The model under review builds one solid part; all positions refer to its coordinate system, in mm. A direction names the side the tool comes from. Coordinates: 2 decimals unless noted, no trailing zeros. Write each loop counter-clockwise with the first axis right and the second up, starting at its lowest first coordinate (ties: lowest second). Pieces come first, ordered by that corner, then holes. Notation, with made-up numbers: (49, -31) - (82, -31) arc R19 ccw to (82, -16) - close; hole circle Ø11 at (8, -15.75). An arc over 180 degrees is marked (long way). Return JSON: item names as keys, results as strings. Group by question number.
(1) For pin 1 Ø4 at (y, z) = (15.5, -5) entering from -X; pin 2 Ø1.5 at (y, z) = (12, -19) entering from -X; pin 3 Ø1 at (x, z) = (8.5, -21.5) entering from -Y, all flat-tipped, find the tip position at first contact; note any pin that passes through.
(2) We need section A-A on z = 7.7. State the section outline as (x, y) points.
(3) Draft analysis for pull direction Z (two halves, no side actions). For faces 4 (the face through (3.46, -10.73, 9.9)), 5 (the face through (0.867, -3.905, -37.042)), 6 (the face through (-1.57, 10.609, 11.487)), 7 (the face through (0, 0, 0)), state which applies: released by +Z, released by -Z, zero draft, split by the parting line, or undercut.
(4) To check wall thickness, follow L1, parallel to Z at x = -4, y = 2; L2, parallel to X at y = 9.75, z = 7.7; L3, parallel to X at y = -10.5, z = 7.7. State the ranges of each line that lie inside material, in increasing order. Write a range as from..to.
(5) Tool access review of faces 1 (the face through (-6.92, 13.31, 7.49)), 2 (the face through (4, -7, 15.2)), 3 (the face through (0, 0, -34)): name each direction out of +Z, -Z, +X, -X, +Y, -Y from which nothing blocks a thin tool from reaching the whole face with its end or side.
```python
from build123d import *

# Parameters (mm, degrees)
SKETCH_1_R               = 15
SKETCH_1_R_2             = 7.55
EXTRUDE_1_DEPTH          = 15.2
CUT_EXTRUDE_1_DEPTH      = 27.096743092
CUT_EXTRUDE_1_DEPTH_BACK = 27.096743092
SKETCH_2_R               = 4.1
SKETCH_8_R               = 4
CUT_EXTRUDE_2_DEPTH      = 6


with BuildPart() as part:
    # 스케치1 → 보스-돌출1 (new body)
    with BuildSketch(Plane.XY):
        with Locations(Location((0, 0, 0), (0, 0, 180))):
            Circle(SKETCH_1_R)
        with Locations(Location((0, 0, 0), (0, 0, 180))):
            Circle(SKETCH_1_R_2, mode=Mode.SUBTRACT)
    extrude(amount=EXTRUDE_1_DEPTH)

    # 스케치2 → 컷-돌출1 (cut, two sides: drawn at the far end of the back side and taken through both)
    with BuildSketch(Plane(origin=(0, 0, 0), x_dir=(1, 0, 0), z_dir=(0, 1, 0)).offset(-CUT_EXTRUDE_1_DEPTH_BACK)):
        with Locations(Location((0, -7.7, 0), (0, 0, 270))):
            Circle(SKETCH_2_R)
    extrude(amount=CUT_EXTRUDE_1_DEPTH + CUT_EXTRUDE_1_DEPTH_BACK, mode=Mode.SUBTRACT)

    # 스케치3 for 로프트4 → 로프트4 section 0
    with BuildSketch(Plane.XY):
        with BuildLine():
            # circular arc as an exact rational Bezier (weights 1, cos(half-angle), 1)
            Bezier((8, -13.856406461), (16.000000001, -9.237604308), (16, 0), weights=[1, 0.866025404, 1])
            Bezier((16, 0), (16.000000001, 9.237604308), (8, 13.856406461), weights=[1, 0.866025404, 1])
            Bezier((8, 13.856406461), (0, 18.475208613), (-8, 13.856406461), weights=[1, 0.866025404, 1])
            Bezier((-8, 13.856406461), (-16.000000001, 9.237604308), (-16, 0), weights=[1, 0.866025404, 1])
            Bezier((-16, 0), (-16.000000001, -9.237604308), (-8, -13.856406461), weights=[1, 0.866025404, 1])
            Bezier((-8, -13.856406461), (0, -18.475208613), (8, -13.856406461), weights=[1, 0.866025404, 1])
        make_face()
    # 스케치4 → 로프트4 section 1
    with BuildSketch(Plane.XY.offset(-15)):
        with BuildLine():
            Line((11.25, -19.485571585), (22.5, 0))
            Line((22.5, 0), (11.25, 19.485571585))
            Line((11.25, 19.485571585), (-11.25, 19.485571585))
            Line((-11.25, 19.485571585), (-22.5, 0))
            Line((-22.5, 0), (-11.25, -19.485571585))
            Line((-11.25, -19.485571585), (11.25, -19.485571585))
        make_face()
    loft()

    # 로프트5: read off the stored shape, not the designer's step
    # 로프트5: loft between two sections, ruled curve by curve
    loft_5_from = [
        Edge.make_bspline([(22.5, 0, -15), (20.625, -3.247595264, -15), (18.75, -6.495190528, -15), (15, -12.990381057, -15), (13.125, -16.237976321, -15), (11.25, -19.485571585, -15)], [0, 0, 0, 0, 0.5, 0.5, 1, 1, 1, 1], 3),
        Edge.make_bspline([(11.25, -19.485571585, -15), (7.5, -19.485571585, -15), (3.75, -19.485571585, -15), (-3.75, -19.485571585, -15), (-7.5, -19.485571585, -15), (-11.25, -19.485571585, -15)], [0, 0, 0, 0, 0.5, 0.5, 1, 1, 1, 1], 3),
        Edge.make_bspline([(11.25, 19.485571585, -15), (13.125, 16.237976321, -15), (15, 12.990381057, -15), (18.75, 6.495190528, -15), (20.625, 3.247595264, -15), (22.5, 0, -15)], [0, 0, 0, 0, 0.5, 0.5, 1, 1, 1, 1], 3),
        Edge.make_bspline([(-11.25, -19.485571585, -15), (-13.125, -16.237976321, -15), (-15, -12.990381057, -15), (-18.75, -6.495190528, -15), (-20.625, -3.247595264, -15), (-22.5, 0, -15)], [0, 0, 0, 0, 0.5, 0.5, 1, 1, 1, 1], 3),
        Edge.make_bspline([(-22.5, 0, -15), (-20.625, 3.247595264, -15), (-18.75, 6.495190528, -15), (-15, 12.990381057, -15), (-13.125, 16.237976321, -15), (-11.25, 19.485571585, -15)], [0, 0, 0, 0, 0.5, 0.5, 1, 1, 1, 1], 3),
        Edge.make_bspline([(-11.25, 19.485571585, -15), (-7.5, 19.485571585, -15), (-3.75, 19.485571585, -15), (3.75, 19.485571585, -15), (7.5, 19.485571585, -15), (11.25, 19.485571585, -15)], [0, 0, 0, 0, 0.5, 0.5, 1, 1, 1, 1], 3),
    ]
    loft_5_to = [
        Edge.make_bspline([(5.352991825, 3.333635602, -40), (5.388078026, 2.283194817, -40), (5.423164227, 1.232754033, -40), (5.493336629, -0.868127536, -40), (5.52842283, -1.918568321, -40), (5.563509031, -2.969009106, -40)], [0, 0, 0, 0, 0.5, 0.5, 1, 1, 1, 1], 3),
        Edge.make_bspline([(5.563509031, -2.969009106, -40), (4.671343726, -3.524615039, -40), (3.779178422, -4.080220973, -40), (1.994847814, -5.19143284, -40), (1.10268251, -5.747038774, -40), (0.210517206, -6.302644707, -40)], [0, 0, 0, 0, 0.5, 0.5, 1, 1, 1, 1], 3),
        Edge.make_bspline([(-0.210517206, 6.302644707, -40), (0.716734299, 5.807809856, -40), (1.643985804, 5.312975006, -40), (3.498488815, 4.323305304, -40), (4.42574032, 3.828470453, -40), (5.352991825, 3.333635602, -40)], [0, 0, 0, 0, 0.5, 0.5, 1, 1, 1, 1], 3),
        Edge.make_bspline([(0.210517206, -6.302644707, -40), (-0.716734299, -5.807809856, -40), (-1.643985804, -5.312975006, -40), (-3.498488815, -4.323305304, -40), (-4.42574032, -3.828470453, -40), (-5.352991825, -3.333635602, -40)], [0, 0, 0, 0, 0.5, 0.5, 1, 1, 1, 1], 3),
        Edge.make_bspline([(-5.352991825, -3.333635602, -40), (-5.388078026, -2.283194817, -40), (-5.423164227, -1.232754033, -40), (-5.493336629, 0.868127536, -40), (-5.52842283, 1.918568321, -40), (-5.563509031, 2.969009106, -40)], [0, 0, 0, 0, 0.5, 0.5, 1, 1, 1, 1], 3),
        Edge.make_bspline([(-5.563509031, 2.969009106, -40), (-4.671343726, 3.524615039, -40), (-3.779178422, 4.080220973, -40), (-1.994847814, 5.19143284, -40), (-1.10268251, 5.747038774, -40), (-0.210517206, 6.302644707, -40)], [0, 0, 0, 0, 0.5, 0.5, 1, 1, 1, 1], 3),
    ]
    loft_5 = Solid(Shell([*[Face.make_surface_from_curves(loft_5_from[k], loft_5_to[k]) for k in range(6)], Face(Wire(loft_5_from)), Face(Wire(loft_5_to))]))
    add(loft_5)

    # 스케치8 → 컷-돌출2 (cut)
    with BuildSketch(Plane(origin=(0, 0, -40), x_dir=(-1, 0, 0), z_dir=(0, 0, -1))):
        Circle(SKETCH_8_R)
    extrude(amount=-CUT_EXTRUDE_2_DEPTH, mode=Mode.SUBTRACT)


solid = part.part
```
Ans:
{
 "1": {"pin 1": "x = -11.49", "pin 2": "x = -13.59", "pin 3": "y = -15.58"},
 "2": {"outline": "(-4.1, -14.43) - (-4.1, -6.34) arc R7.55 cw to (-4.1, 6.34) - (-4.1, 14.43) arc R15 ccw to start; (4.1, -14.43) arc R15 ccw to (4.1, 14.43) - (4.1, 6.34) arc R7.55 cw to (4.1, -6.34) - close"},
 "3": {"face 4": "undercut", "face 5": "zero draft", "face 6": "undercut", "face 7": "released by +Z"},
 "4": {"L1": "-40..0", "L2": "-11.4..-4.1, 4.1..11.4", "L3": "-10.71..-4.1, 4.1..10.71"},
 "5": {"face 1": "+Z", "face 2": "+Z, +X, -X, +Y, -Y", "face 3": "-Z"}
}
